Input: part model. Units: mm. Frame: model coordinates. Coordinates: 2 decimals unless noted, no trailing zeros. Order: outer loops, then holes, each group sorted by start corner. A loop starts at its lowest first (then second) coordinate and runs counter-clockwise, first axis right, second up. Notation, with made-up numbers: M -3,-36.75 L 53,-36.75 A14 ccw 53,-13.75 Z; hole C 34,-5.75 d10. An arc over 180 degrees is marked long. One line per item, written item: value.
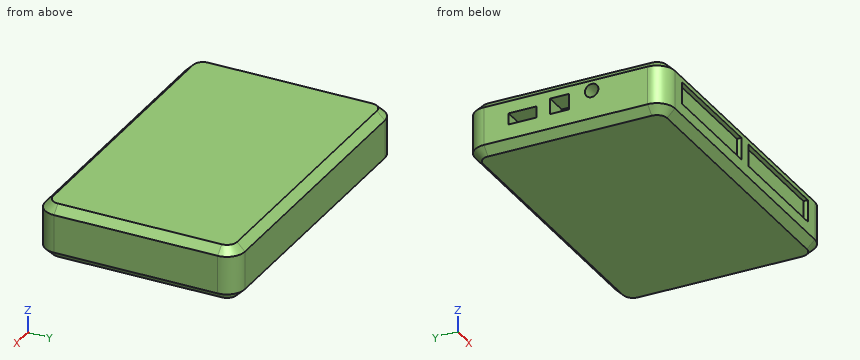
```python
from build123d import *

# Parameters (mm, degrees)
SKETCH1_W           = 137
SKETCH1_H           = 89
BOSS_EXTRUDE1_DEPTH = 24
FILLET2_R           = 8
CHAMFER2_SIZE       = 3.5
SKETCH2_W           = 51.5
SKETCH2_H           = 9.8
CUT_EXTRUDE1_DEPTH  = 2
SKETCH3_R           = 3
SKETCH3_W           = 5
SKETCH3_H           = 12.5
SKETCH3_W_2         = 7
SKETCH3_H_2         = 8.5
CUT_EXTRUDE2_DEPTH  = 10


with BuildPart() as part:
    # Sketch1 → Boss-Extrude1 (new body)
    with BuildSketch(Plane.XY):
        Rectangle(SKETCH1_W, SKETCH1_H)
    extrude(amount=BOSS_EXTRUDE1_DEPTH)

    # Fillet2
    fillet2_edges = [part.edges().sort_by_distance(p)[0] for p in [
        (-68.5, 44.5, 12),
        (68.5, 44.5, 12),
        (68.5, -44.5, 12),
        (-68.5, -44.5, 12),
    ]]
    fillet(fillet2_edges, radius=FILLET2_R)

    # Chamfer2
    chamfer2_edges = [part.edges().sort_by_distance(p)[0] for p in [
        (0, 44.5, 0),
        (0, 44.5, 24),
        (-68.5, 0, 0),
        (68.5, 0, 0),
        (0, -44.5, 0),
        (-66.156854249, 42.156854249, 0),
        (-66.156854249, -42.156854249, 0),
        (66.156854249, -42.156854249, 0),
        (66.156854249, 42.156854249, 0),
        (68.5, 0, 24),
        (-68.5, 0, 24),
        (0, -44.5, 24),
        (-66.156854249, 42.156854249, 24),
        (-66.156854249, -42.156854249, 24),
        (66.156854249, -42.156854249, 24),
        (66.156854249, 42.156854249, 24),
    ]]
    chamfer(chamfer2_edges, length=CHAMFER2_SIZE)

    # Sketch2 → Cut-Extrude1 (cut)
    with BuildSketch(Plane.XZ.offset(44.5)):
        with Locations((-28.75, 13.5)):
            Rectangle(SKETCH2_W, SKETCH2_H)
        with Locations((28.75, 13.5)):
            Rectangle(SKETCH2_W, SKETCH2_H)
    extrude(amount=-CUT_EXTRUDE1_DEPTH, mode=Mode.SUBTRACT)

    # Sketch3 → Cut-Extrude2 (cut)
    with BuildSketch(Plane.ZY.offset(68.5)):
        with Locations((16, -11.5)):
            Circle(SKETCH3_R)
        with Locations((12.5, 19.25)):
            Rectangle(SKETCH3_W, SKETCH3_H)
        with Locations((13.5, 2.75)):
            Rectangle(SKETCH3_W_2, SKETCH3_H_2)
    extrude(amount=-CUT_EXTRUDE2_DEPTH, mode=Mode.SUBTRACT)


solid = part.part
```
(1) First-contact query: pin 1 (3 mm diameter, centred on x = 17.5, z = 14.5, fed in from -Y); pin 2 (0.6 mm diameter, centred on y = -44, z = 14, fed in from +X); pin 3 (2 mm diameter, centred on y = -43.5, z = 14.5, fed in from +X). Flat tips, straight axial feed; report the tip coordinate or a pass-through.
Data:
pin 1: stops at y = -42.5
pin 2: stops at x = 63.99
pin 3: stops at x = 65.79
(2) Ray query, line 1 (Y direction, x = -61.25, z = 16); line 2 (Y direction, x = -63.5, z = 16); line 3 (Z direction, x = -63, y = 21.5). Return the intervals inside material, ascending. Write a range as from..to.
Data:
line 1: y = -44.46..-14.5, -8.5..-1.5, 7..44.46
line 2: y = -43.92..-14.5, -8.5..-1.5, 7..43.92
line 3: z = 0..10, 15..24
(3) Cut plane B-B on y = -11.5. Output: boundary loops of the cut face in (x, z), plus the area to 3 significant figures.
Data:
outline: M -68.5,3.5 L -65,0 L 65,0 L 68.5,3.5 L 68.5,20.5 L 65,24 L -65,24 L -68.5,20.5 L -68.5,19 L -58.5,19 L -58.5,13 L -68.5,13 Z
area: 3,200 mm2
(4) Cut plane A-A on x = 14. Output: boundary loops of the cut face in (y, z), plus the area to 3 significant figures.
Data:
outline: M -44.5,3.5 L -41,0 L 41,0 L 44.5,3.5 L 44.5,20.5 L 41,24 L -41,24 L -44.5,20.5 L -44.5,18.4 L -42.5,18.4 L -42.5,8.6 L -44.5,8.6 Z
area: 2,090 mm2
